```python
from build123d import *

# Parameters (mm, degrees)
F1_DEPTH = 25.4


with BuildPart() as f1:
    # F0 (on Front) → F1 (new body)
    with BuildSketch(Plane.XZ):
        Polygon((13.867266, 38.1), (0, 38.1), (-13.867266, 38.1), (-35.11315, 20.272587), (-39.929201, -7.040595), (-26.061935, -31.059405), (0, -40.545173), (26.061935, -31.059405), (39.929201, -7.040595), (35.11315, 20.272587), align=None)
        Polygon((-9.244844, 25.4), (0, 25.4), (9.244844, 25.4), (23.408767, 13.515058), (26.619467, -4.69373), (17.374623, -20.70627), (0, -27.030115), (-17.374623, -20.70627), (-26.619467, -4.69373), (-23.408767, 13.515058), align=None, mode=Mode.SUBTRACT)
    extrude(amount=F1_DEPTH)


solid = f1.part
```
Geometry check sheet. Reference: the model listing, model coordinates, mm. A direction names the side the tool comes from. Give positions to 0.01 mm unless a question says otherwise; leave off trailing zeros. Order: outer loops, then holes, each group sorted by start corner. A loop starts at its lowest first (then second) coordinate and runs counter-clockwise, first axis right, second up.
1. Gauge pin test, flat ends, axial feed: pin 1 Ø3 at (x, y) = (17.5, -11.5) entering from -Z; pin 2 Ø6 at (x, y) = (13.5, -13.5) entering from -Z; pin 3 Ø4 at (y, z) = (-23, 16.5) entering from -X. Record the tip position at first contact, or that the pin passes through.
2. Release check for a two-part mould opening along X. For faces 3 (the face through (-24.34, -12.52, 29.31)), 4 (the face through (22.06, -12.52, -12.59)), 5 (the face through (12.85, -12.52, -35.87)), 6 (the face through (0, -13, 38.1)) record: pulls with the +X half, pulls with the -X half, needs draft (parallel to the pull), parting line crosses it, or undercut.
3. Section check B-B, the plane x = -5.5. Enter the section's corners in (y, z), and give its area (3 significant figures).
4. Section check A-A, the plane y = -7.5. Enter the section's corners in (x, z).
5. Thickness scan on L1, parallel to Z at x = 18, y = -6; L2, parallel to X at y = -22.5, z = -10; L3, parallel to X at y = -16, z = 14.5. Record the ranges inside material, lowest first.
6. Section check C-C, the plane z = -16. Enter the section's corners in (x, y).
7. Access from +Z, -Z, +X, -X, +Y, -Y to the whole of each face (thin tool, end or side, straight path). Record for faces 1 (the face through (8.809, -12.522, -23.824)), 2 (the face through (37.555, -12.522, 6.425)).
Values follow:
1. pin 1: stops at z = -34.72
1. pin 2: stops at z = -36.72
1. pin 3: stops at x = -36.13
2. face 3: pulls with the -X half
2. face 4: undercut
2. face 5: pulls with the +X half
2. face 6: needs draft
3. outline: (-25.4, -38.54) - (0, -38.54) - (0, -25.03) - (-25.4, -25.03) - close; (-25.4, 25.4) - (0, 25.4) - (0, 38.1) - (-25.4, 38.1) - close
3. area: 666 mm2
4. outline: (-39.93, -7.04) - (-26.06, -31.06) - (0, -40.55) - (26.06, -31.06) - (39.93, -7.04) - (35.11, 20.27) - (13.87, 38.1) - (-13.87, 38.1) - (-35.11, 20.27) - close; hole (-26.62, -4.69) - (-17.37, -20.71) - (0, -27.03) - (17.37, -20.71) - (26.62, -4.69) - (23.41, 13.52) - (9.24, 25.4) - (-9.24, 25.4) - (-23.41, 13.52) - close
5. L1: z = -33.99 to -19.62, 18.05 to 34.63
5. L2: x = -38.22 to -23.56, 23.56 to 38.22
5. L3: x = -36.13 to -22.23, 22.23 to 36.13
6. outline: (-34.76, -25.4) - (-20.09, -25.4) - (-20.09, 0) - (-34.76, 0) - close; (20.09, -25.4) - (34.76, -25.4) - (34.76, 0) - (20.09, 0) - close
7. face 1: +Y, -Y
7. face 2: +Z, +X, +Y, -Y
